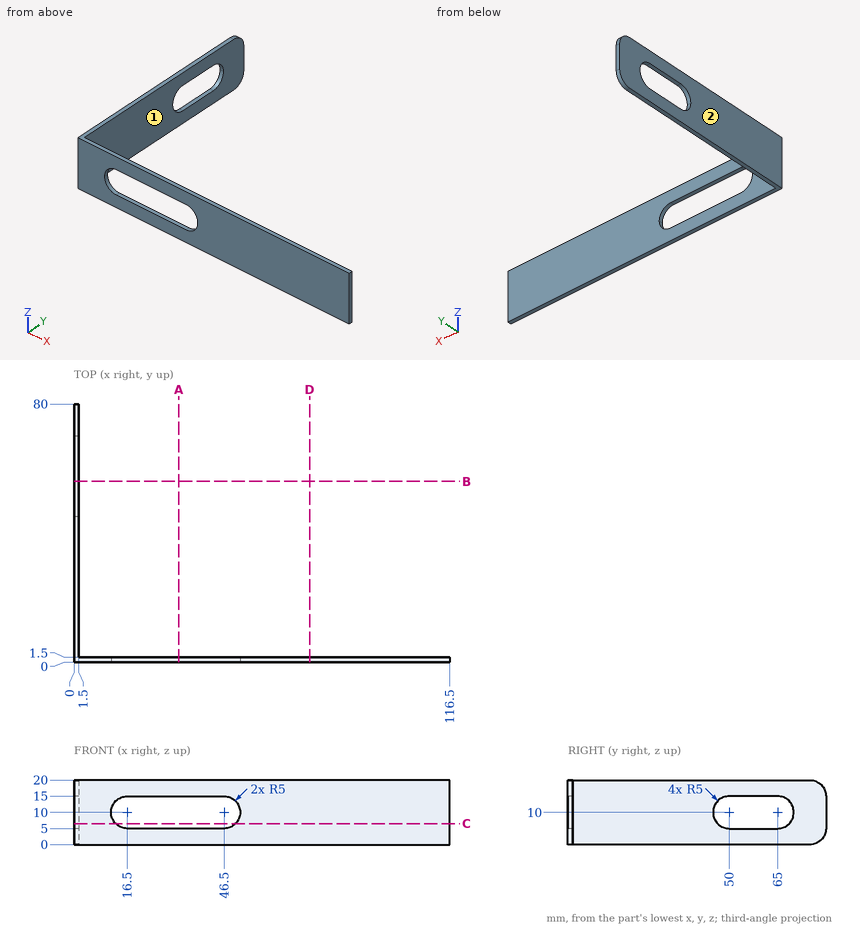
Source: three-view drawing plus pictorial views. Frame: mm from the lowest corner of the part. A direction names the side the tool comes from. Round coordinates to 2 decimals unless told otherwise and drop trailing zeros. Loops run counter-clockwise (first coordinate to the right, second up) from the corner with the lowest first, then second, coordinate; pieces in that order, holes last.
Q1. Ray query, line 1 (Y direction, x = 72, z = 18.75). Return the intervals inside material, ascending.
Q2. Access query for the marked faces 1 and 2. Directions: +Z, -Z, +X, -X, +Y, -Y. A direction counts if a zero-diameter tool reaches every point of the face in a straight line with its end or side. Return the directions, or none.
Q3. First-contact query: P1, Ø10, axis at y = 51, z = 9, coming from the +X side; P2, Ø2, axis at x = 15.5, z = 16.5, coming from the +Y side. Flat tips, straight axial feed; report the tip coordinate or a pass-through.
Q4. Section C-C, the plane z = 6.5. Return loops of the section in (x, y), plus the area to 3 significant figures.
Q5. Section D-D, the plane x = 73. Return loops of the section in (y, z).
Q6. Section A-A, the plane x = 32.5. Return loops of the section in (y, z).
Solutions:
1. line 1: y = 0 to 1.5
2. face 1: +Z, -Z, +X, +Y
2. face 2: +Z, -Z, -X, +Y, -Y
3. P1: stops at x = 1.5
3. P2: stops at y = 1.5
4. outline: (0, 0) - (12.93, 0) - (12.93, 1.5) - (1.5, 1.5) - (1.5, 46.43) - (0, 46.43) - close; (0, 68.57) - (1.5, 68.57) - (1.5, 80) - (0, 80) - close; (50.07, 0) - (116.5, 0) - (116.5, 1.5) - (50.07, 1.5) - close
4. area: 204 mm2
5. outline: (0, 0) - (1.5, 0) - (1.5, 20) - (0, 20) - close
6. outline: (0, 0) - (1.5, 0) - (1.5, 5) - (0, 5) - close; (0, 15) - (1.5, 15) - (1.5, 20) - (0, 20) - close
